from build123d import *

# Parameters (mm, degrees)
SKETCH1_W           = 25.4
SKETCH1_H           = 304.8
BOSS_EXTRUDE1_DEPTH = 25.4
SKETCH2_W           = 20.32
SKETCH2_H           = 22.86
CUT_EXTRUDE1_DEPTH  = 307.909367729
SKETCH3_R           = 9.525
BOSS_EXTRUDE2_DEPTH = 2.54
SKETCH4_W           = 25.4
SKETCH4_H           = 25.4
BOSS_EXTRUDE3_DEPTH = 127
SKETCH5_W           = 20.32
SKETCH5_H           = 22.86
CUT_EXTRUDE2_DEPTH  = 127
SKETCH6_R           = 3.175
CUT_EXTRUDE3_DEPTH  = 12.7
CUT_EXTRUDE4_START  = -12.7
SKETCH7_R           = 3.175
CUT_EXTRUDE4_DEPTH  = 12.7


with BuildPart() as part:
    # Sketch1 → Boss-Extrude1 (new body)
    with BuildSketch(Plane(origin=(0, 0, 0), x_dir=(1, 0, 0), z_dir=(0, 1, 0))):
        with Locations((12.7, 152.4)):
            Rectangle(SKETCH1_W, SKETCH1_H)
    extrude(amount=BOSS_EXTRUDE1_DEPTH)

    # Sketch2 → Cut-Extrude1 (cut, through all)
    with BuildSketch(Plane.XY):
        with Locations((12.7, 11.43)):
            Rectangle(SKETCH2_W, SKETCH2_H)
    extrude(amount=-CUT_EXTRUDE1_DEPTH, mode=Mode.SUBTRACT)

    # Sketch3 → Boss-Extrude2 (add)
    with BuildSketch(Plane(origin=(0, 25.4, 0), x_dir=(1, 0, 0), z_dir=(0, 1, 0))):
        with Locations(Location((12.7, 12.7, 0), (0, 0, 90))):
            Circle(SKETCH3_R)
        with Locations(Location((12.7, 292.1, 0), (0, 0, 90))):
            Circle(SKETCH3_R)
    extrude(amount=BOSS_EXTRUDE2_DEPTH)

    # Sketch4 → Boss-Extrude3 (add)
    with BuildSketch(Plane(origin=(25.4, 0, 0), x_dir=(0, 0, -1), z_dir=(1, 0, 0))):
        with Locations((228.6, 12.7)):
            Rectangle(SKETCH4_W, SKETCH4_H)
    extrude(amount=BOSS_EXTRUDE3_DEPTH)

    # Sketch5 → Cut-Extrude2 (cut)
    with BuildSketch(Plane(origin=(152.4, 0, 0), x_dir=(0, 0, -1), z_dir=(1, 0, 0))):
        with Locations((228.6, 11.43)):
            Rectangle(SKETCH5_W, SKETCH5_H)
    extrude(amount=-CUT_EXTRUDE2_DEPTH, mode=Mode.SUBTRACT)

    # Mirror5: part across plane


with BuildPart() as part_1:
    add(part.part)
    add(part.part.mirror(Plane.ZY.offset(-152.4)))

    # Sketch6 → Cut-Extrude3 (cut)
    with BuildSketch(Plane(origin=(304.8, 0, 0), x_dir=(0, 0, -1), z_dir=(1, 0, 0))):
        with Locations((12.7, 12.7)):
            Circle(SKETCH6_R)
        with Locations((292.1, 12.7)):
            Circle(SKETCH6_R)
    extrude(amount=-CUT_EXTRUDE3_DEPTH, mode=Mode.SUBTRACT)

    # Sketch7 → Cut-Extrude4 (cut)
    with BuildSketch(Plane.ZY.offset(CUT_EXTRUDE4_START)):
        with Locations(Location((-292.1, 12.7, 0), (0, 0, 180))):
            Circle(SKETCH7_R)
        with Locations(Location((-12.7, 12.7, 0), (0, 0, 180))):
            Circle(SKETCH7_R)
    extrude(amount=CUT_EXTRUDE4_DEPTH, mode=Mode.SUBTRACT)


solid = part_1.part
Build history of the part. All positions in model axes, mm. A direction names the side the tool comes from. Round coordinates to 2 decimals unless told otherwise and drop trailing zeros. Write each loop counter-clockwise with the first axis right and the second up, starting at its lowest first coordinate (ties: lowest second). Pieces come first, ordered by that corner, then holes. Notation, with made-up numbers: M 17,10 L 60,10 A26 cw 60,26 Z; hole C -39,55.25 d5. An arc over 180 degrees is marked long. Use CSV: the item, a comma, the result in double quotes.
1. Tool access for faces 1 (the face through (25.4, 13, -273)), 2 (the face through (302.26, 11, -150)), 3 (the face through (6.26, 26.65, -5.68)): list every direction of +Z, -Z, +X, -X, +Y, -Y with a clear straight run to the whole face (end or side of a thin tool).
Reply:
face 1,"-Z, +Y, -Y"
face 2,"+Z, -Z, -Y"
face 3,"+Y"
2. Wall check: probe 1 along X at (y, z) = (4, -221); probe 2 along Z at (x, y) = (1, 12.7) (3 decimals); probe 3 along Y at (x, z) = (1, -292). Give the ranges that are in metal, low to high. Write a range as from..to.
Reply:
probe 1,"x = 0..2.54, 22.86..25.4, 279.4..281.94, 302.26..304.8"
probe 2,"z = -304.8..-295.275, -288.925..-15.875, -9.525..0"
probe 3,"y = 0..9.53, 15.87..25.4"
3. Flat gauge pins, fed straight in: pin 1 (4 mm diameter, centred on y = 12.7, z = -12.7, fed in from -X); pin 2 (10 mm diameter, centred on x = 208, z = -225, fed in from -Y); pin 3 (5 mm diameter, centred on x = 43.5, y = 24, fed in from +Z). Where does each tip first touch, or does it go through?
Reply:
pin 1,"stops at x = 22.86"
pin 2,"stops at y = 22.86"
pin 3,"stops at z = -215.9"
4. Saw through at A-A (z = -262.5). Give the cut face in (x, y).
Reply:
outline,"M 0,0 L 2.54,0 L 2.54,22.86 L 22.86,22.86 L 22.86,0 L 25.4,0 L 25.4,25.4 L 0,25.4 Z; M 279.4,0 L 281.94,0 L 281.94,22.86 L 302.26,22.86 L 302.26,0 L 304.8,0 L 304.8,25.4 L 279.4,25.4 Z"
5. Saw through at B-B (x = 37). Give the cut face in (y, z).
Reply:
outline,"M 0,-241.3 L 25.4,-241.3 L 25.4,-215.9 L 0,-215.9 L 0,-218.44 L 22.86,-218.44 L 22.86,-238.76 L 0,-238.76 Z"
6. Saw through at C-C (z = -223.5). Give the cut face in (x, y).
Reply:
outline,"M 0,0 L 2.54,0 L 2.54,22.86 L 22.86,22.86 L 22.86,0 L 25.4,0 L 25.4,22.86 L 279.4,22.86 L 279.4,0 L 281.94,0 L 281.94,22.86 L 302.26,22.86 L 302.26,0 L 304.8,0 L 304.8,25.4 L 0,25.4 Z"
7. Two-plate mould, pull along Z, no slides. Class faces 4 (the face through (292, 22.86, -150)), 5 (the face through (151, 11, -218.44)), 6 (the face through (25.4, 12, -228)), 7 (the face through (154, 13, -241.3)): +Z half, -Z half, draft (parallel to the pull), parting line (faces both ways), or undercut.
Reply:
face 4,"draft"
face 5,"undercut"
face 6,"undercut"
face 7,"-Z half"
